For this review, take the finished solid that the model builds, in its own axes (mm). Round coordinates to 2 decimals unless told otherwise and drop trailing zeros. Order: outer loops, then holes, each group sorted by start corner. A loop starts at its lowest first (then second) coordinate and runs counter-clockwise, first axis right, second up. Notation, with made-up numbers: M 85,47 L 117,47 A22 ccw 117,84 Z; hole C -34.5,-9 d4. An arc over 180 degrees is marked long. Answer as a JSON object with one key per item and string values.
from build123d import *

# Parameters (mm, degrees)
F3_DEPTH = 20.001
F4_R     = 10
F5_DEPTH = 20.0010001


with BuildPart() as f1:
    # F0 (on Front) → F1 (revolve)
    with BuildSketch(Plane.XZ):
        Polygon((-4.2, 0), (-4.2, 20), (-24.2264973081, 20), (-35.7735026919, 0), align=None)
    revolve(axis=Axis((0, 0, 10), (0, 0, 1)))

    # F2 (on Top) → F3 (cut, through all)
    with BuildSketch(Plane.XY):
        with BuildLine():
            ThreePointArc((-17.2168920075, 31.3579674795), (0, 24.2264973081), (17.2168920075, 31.3579674795))
            ThreePointArc((17.2168920075, 31.3579674795), (0, 35.7735026919), (-17.2168920075, 31.3579674795))
        make_face()
        with BuildLine():
            ThreePointArc((31.3579674795, -17.2168920075), (34.6520405524, -8.887045651), (35.7735026919, 0))
            ThreePointArc((35.7735026919, 0), (34.6520405524, 8.887045651), (31.3579674795, 17.2168920075))
            ThreePointArc((31.3579674795, 17.2168920075), (24.2264973081, 0), (31.3579674795, -17.2168920075))
        make_face()
        with BuildLine():
            ThreePointArc((-17.2168920075, -31.3579674795), (0, -35.7735026919), (17.2168920075, -31.3579674795))
            ThreePointArc((17.2168920075, -31.3579674795), (0, -24.2264973081), (-17.2168920075, -31.3579674795))
        make_face()
        with BuildLine():
            ThreePointArc((-31.3579674795, -17.2168920075), (-24.2264973081, 0), (-31.3579674795, 17.2168920075))
            ThreePointArc((-31.3579674795, 17.2168920075), (-35.7735026919, 0), (-31.3579674795, -17.2168920075))
        make_face()
    extrude(amount=F3_DEPTH, mode=Mode.SUBTRACT)

    # F4 (on Top) → F5 (cut, through all)
    with BuildSketch(Plane.XY):
        with Locations((-12.6478431701, -12.6478431701)):
            Circle(F4_R)
        with Locations((12.6478431701, -12.6478431701)):
            Circle(F4_R)
        with Locations((12.6478431701, 12.6478431701)):
            Circle(F4_R)
        with Locations((-12.6478431701, 12.6478431701)):
            Circle(F4_R)
    extrude(amount=F5_DEPTH, mode=Mode.SUBTRACT)


solid = f1.part
1) Add section A-A on z = 18.75. State the section outline as (x, y) points, and give its area (3 significant figures).
Geometry check:
{"outline": "M -24.59,-4.2 A24.95 ccw -22.48,-10.82 A10 cw long -10.82,-22.48 A24.95 ccw -4.2,-24.59 A24.35 cw 4.2,-24.59 A24.95 ccw 10.82,-22.48 A10 cw long 22.48,-10.82 A24.95 ccw 24.59,-4.2 A24.35 cw 24.59,4.2 A24.95 ccw 22.48,10.82 A10 cw long 10.82,22.48 A24.95 ccw 4.2,24.59 A24.35 cw -4.2,24.59 A24.95 ccw -10.82,22.48 A10 cw long -22.48,10.82 A24.95 ccw -24.59,4.2 A24.35 cw Z; hole C 0,0 d8.4", "area": "766 mm²"}
2) Mouldability with a two-part tool opening along Y and no side actions: class faces 1 (the flat face through (0, -5, 20)), 2 (the conical face through (-21.5, -21.04, 9.86)), 3 (the cylindrical face through (4.712, 6.563, 9.86)) as +Y half, -Y half, draft (parallel to the pull), parting line (faces both ways), or undercut.
Geometry check:
{"face 1": "draft", "face 2": "-Y half", "face 3": "undercut"}
3) Add section B-B on z = 8.5. State the section outline as (x, y) points, and give its area (3 significant figures).
Geometry check:
{"outline": "M -27.99,-13.01 A30.87 ccw -13.01,-27.99 A24.35 cw 13.01,-27.99 A30.87 ccw 27.99,-13.01 A24.35 cw 27.99,13.01 A30.87 ccw 13.01,27.99 A24.35 cw -13.01,27.99 A30.87 ccw -27.99,13.01 A24.35 cw Z; hole C -12.65,-12.65 d20; hole C -12.65,12.65 d20; hole C 0,0 d8.4; hole C 12.65,-12.65 d20; hole C 12.65,12.65 d20", "area": "1,210 mm²"}
4) Add section C-C on y = -14. State how many separate pieces and enclosed holes the cut face has, and give its area (3 significant figures).
Geometry check:
{"separate pieces": "3", "enclosed holes": "0", "area": "249 mm²"}
5) Insertion check: P1, Ø6, axis at y = 14, z = 3.5, coming from the -X side; P2, Ø2, axis at y = 0.5, z = 15, coming from the -X side; P3, Ø4, axis at x = 1, z = 12.5, coming from the +Y side. Each pin has a flat end and moves straight along its axis. Give the tip position at first contact, or say it passes through.
Geometry check:
{"P1": "stops at x = -30.62", "P2": "stops at x = -24.27", "P3": "stops at y = 24.41"}
6) For L1, parallel to Y at x = 0, z = 16; L2, parallel to X at y = 11, z = 6; L3, parallel to Y at x = -13.5, z = 7.5, list the stretches that pass through material, from the lowest coordinate up.
Geometry check:
{"L1": "y = -24.23 to -4.2, 4.2 to 24.23", "L2": "x = -26.85 to -22.51, -2.78 to 2.78, 22.51 to 26.85", "L3": "y = -28.31 to -22.61, -2.68 to 2.68, 22.61 to 28.31"}
